from build123d import *

# Parameters (mm, degrees)
BOSS_EXTRUDE1_DEPTH   = 12.7
BOSS_EXTRUDE1_2_DEPTH = 12.7
BOSS_EXTRUDE2_REACH   = 26.909
CUT_EXTRUDE2_REACH    = 19.991
FILLET1_R             = 6.35
FILLET3_R             = 0.5


with BuildPart() as part:
    # Sketch1 → Boss-Extrude1 (new body)
    with BuildSketch(Plane(origin=(0, 0, 0), x_dir=(0, 0, -1), z_dir=(1, 0, 0))):
        with BuildLine():
            Line((9.214036359, -0.723419074), (9.52014781, -1.005011796))
            Line((9.52014781, -1.005011796), (9.931084378, -1.111282001))
            Line((9.931084378, -1.111282001), (9.790954894, -0.710625106))
            Line((9.790954894, -0.710625106), (9.214036359, -0.17991624))
            Line((9.214036359, -0.17991624), (8.098182028, -0.17991624))
            Line((8.098182028, -0.17991624), (8.098182028, -2.893389425))
            ThreePointArc((8.098182028, -2.893389425), (8.258948932, -3.437161263), (8.68955765, -3.80609207))
            Line((8.68955765, -3.80609207), (10.464036359, -4.600540583))
            Line((10.464036359, -4.600540583), (12.238515069, -3.80609207))
            ThreePointArc((12.238515069, -3.80609207), (12.669123787, -3.437161263), (12.829890691, -2.893389425))
            Line((12.829890691, -2.893389425), (12.829890691, -0.17991624))
            Line((12.829890691, -0.17991624), (11.714036359, -0.17991624))
            Line((11.714036359, -0.17991624), (11.714036359, -2.617334806))
            Line((11.714036359, -2.617334806), (9.214036359, -2.617334806))
            Line((9.214036359, -2.617334806), (9.214036359, -0.723419074))
        make_face()
    extrude(amount=BOSS_EXTRUDE1_DEPTH)


with BuildPart() as body_2:
    # Sketch1 → Boss-Extrude1 2 (new body)
    with BuildSketch(Plane(origin=(0, 0, 0), x_dir=(0, 0, -1), z_dir=(1, 0, 0))):
        with BuildLine():
            Line((-8.098182028, -0.17991624), (-9.214036359, -0.17991624))
            Line((-9.214036359, -0.17991624), (-9.790954894, -0.710625106))
            Line((-9.790954894, -0.710625106), (-9.931084378, -1.111282001))
            Line((-9.931084378, -1.111282001), (-9.52014781, -1.005011796))
            Line((-9.52014781, -1.005011796), (-9.214036359, -0.723419074))
            Line((-9.214036359, -0.723419074), (-9.214036359, -2.617334806))
            Line((-9.214036359, -2.617334806), (-11.714036359, -2.617334806))
            Line((-11.714036359, -2.617334806), (-11.714036359, -0.17991624))
            Line((-11.714036359, -0.17991624), (-12.829890691, -0.17991624))
            Line((-12.829890691, -0.17991624), (-12.829890691, -2.893389425))
            ThreePointArc((-12.829890691, -2.893389425), (-12.669123787, -3.437161263), (-12.238515069, -3.80609207))
            Line((-12.238515069, -3.80609207), (-10.464036359, -4.600540583))
            Line((-10.464036359, -4.600540583), (-8.68955765, -3.80609207))
            ThreePointArc((-8.68955765, -3.80609207), (-8.258948932, -3.437161263), (-8.098182028, -2.893389425))
            Line((-8.098182028, -2.893389425), (-8.098182028, -0.17991624))
        make_face()
    extrude(amount=BOSS_EXTRUDE1_2_DEPTH)

    # Sketch2 → Boss-Extrude2 (add, up to next)
    with BuildSketch(Plane.XY.offset(-8.098182028), mode=Mode.PRIVATE) as boss_extrude2_sk1:
        Polygon((5.47811731, -0.17991624), (7.387826905, -0.17991624), (7.387826905, -1.641579788), (6.432972108, -2.596434586), (5.47811731, -1.641579788), align=None)
    boss_extrude2_tool1 = extrude(boss_extrude2_sk1.sketch, amount=BOSS_EXTRUDE2_REACH, mode=Mode.PRIVATE) - body_2.part

    add(part.part)  # Boss-Extrude2 merges part
    add(boss_extrude2_tool1.solids().sort_by_distance((6.432972, -1.169053, -8.098182))[0])

    # Sketch5 → Loft4 section 0
    with BuildSketch(Plane(origin=(0, -0.17991624, 0), x_dir=(1, 0, 0), z_dir=(0, 1, 0))):
        with BuildLine():
            Line((7.387826905, 4.313769845), (7.387826905, -4.313769845))
            Line((7.387826905, -4.313769845), (6.432972108, -5.268624642))
            Line((6.432972108, -5.268624642), (5.47811731, -4.313769845))
            Line((5.47811731, -4.313769845), (5.47811731, 4.313769845))
            Line((5.47811731, 4.313769845), (6.432972108, 5.268624642))
            Line((6.432972108, 5.268624642), (7.387826905, 4.313769845))
        make_face()
    # Sketch6 → Loft4 section 1
    with BuildSketch(Plane(origin=(0, -10.33991624, 0), x_dir=(1, 0, 0), z_dir=(0, 1, 0))):
        with BuildLine():
            Line((6.432972108, -1.017808112), (5.47811731, -0.062953314))
            Line((5.47811731, -0.062953314), (5.47811731, 0.062953314))
            Line((5.47811731, 0.062953314), (6.432972108, 1.017808112))
            Line((6.432972108, 1.017808112), (7.387826905, 0.062953314))
            Line((7.387826905, 0.062953314), (7.387826905, -0.062953314))
            Line((7.387826905, -0.062953314), (6.432972108, -1.017808112))
        make_face()
    loft()

    # Sketch4 → Cut-Extrude2 (cut, up to next)
    with BuildSketch(Plane.ZY.offset(-5.47811731), mode=Mode.PRIVATE) as cut_extrude2_sk1:
        with BuildLine():
            Line((0.863271786, -3.536832517), (0.455999977, -3.536832517))
            Line((0.455999977, -3.536832517), (0.455999977, -3.028389789))
            Line((0.455999977, -3.028389789), (-0.455999977, -3.028389789))
            Line((-0.455999977, -3.028389789), (-0.455999977, -3.536832517))
            Line((-0.455999977, -3.536832517), (-0.863271786, -3.536832517))
            ThreePointArc((-0.863271786, -3.536832517), (-1.248147381, -3.717660499), (-1.354637866, -4.129349409))
            Line((-1.354637866, -4.129349409), (-0.455999977, -8.902101345))
            Line((-0.455999977, -8.902101345), (-0.455999977, -12.003161214))
            Line((-0.455999977, -12.003161214), (0.455999977, -12.003161214))
            Line((0.455999977, -12.003161214), (0.455999977, -8.902101345))
            Line((0.455999977, -8.902101345), (1.354637866, -4.129349409))
            ThreePointArc((1.354637866, -4.129349409), (1.248147381, -3.717660499), (0.863271786, -3.536832517))
        make_face()
    cut_extrude2_tool1 = extrude(cut_extrude2_sk1.sketch, amount=-CUT_EXTRUDE2_REACH, mode=Mode.PRIVATE) & body_2.part
    add(cut_extrude2_tool1.solids().sort_by_distance((5.478117, -6.679281, 0))[0], mode=Mode.SUBTRACT)

    # Fillet1
    # the kernel refuses this fillet: 6.35 mm, written as the material it adds along each edge
    with BuildSketch(Plane(origin=(11.918265355, 2.888858661, -1.067268312), x_dir=(0.268949751125616, 0.268949751125617, -0.9248416419792839), z_dir=(-0.6539617965672524, -0.6539617965672533, -0.3803523856387155))) as fillet1_piece_1_section:
        with BuildLine():
            CenterArc((FILLET1_R * 0.436389328948, FILLET1_R), FILLET1_R, 222.8481144, 47.1518856)
            Line((-FILLET1_R * 0.296769712888, FILLET1_R * 0.319942782278), (0, 0))
            Line((0, 0), (FILLET1_R * 0.436389328948, 0))
        make_face()
    fillet1_piece_1 = extrude(amount=15.315469113, mode=Mode.PRIVATE)
    fillet1_piece_1 = split(fillet1_piece_1, bisect_by=Plane(origin=(7.387826905, 2.888858661, -1.067268312), z_dir=(-1, 0, 0)), keep=Keep.TOP, mode=Mode.PRIVATE)
    fillet1_piece_1 = fillet1_piece_1 - Plane(origin=(0.404018799, -5.547737398, -6.35885034), x_dir=(0.7071067811865474, 0.7071067811865479, 0), z_dir=(0.6539617965672531, -0.6539617965672526, -0.38035238563871554)) * Cylinder(6.35, 42, mode=Mode.PRIVATE)
    add(fillet1_piece_1)
    with BuildSketch(Plane(origin=(10.963410557, -7.126873035, -6.892543527), x_dir=(-0.26894975112561653, 0.26894975112561653, -0.9248416419792839), z_dir=(-0.6539617965672532, 0.6539617965672525, 0.38035238563871554))) as fillet1_piece_2_section:
        with BuildLine():
            CenterArc((FILLET1_R * 0.436389328948, FILLET1_R), FILLET1_R, 222.8481144, 47.1518856)
            Line((-FILLET1_R * 0.296769712888, FILLET1_R * 0.319942782278), (0, 0))
            Line((0, 0), (FILLET1_R * 0.436389328948, 0))
        make_face()
    fillet1_piece_2 = extrude(amount=15.315469113, mode=Mode.PRIVATE)
    fillet1_piece_2 = split(fillet1_piece_2, bisect_by=Plane(origin=(5.47811731, -7.126873035, -6.892543527), z_dir=(1, 0, 0)), keep=Keep.TOP, mode=Mode.PRIVATE)
    fillet1_piece_2 = fillet1_piece_2 - Plane(origin=(11.012970172, -6.996692643, -7.201580889), x_dir=(-0.707106781186548, 0.7071067811865471, 0), z_dir=(0.6539617965672524, 0.6539617965672532, 0.38035238563871543)) * Cylinder(6.35, 42, mode=Mode.PRIVATE)
    add(fillet1_piece_2)
    with BuildSketch(Plane(origin=(1.902533659, -7.126873035, 6.892543527), x_dir=(0.33552051071253974, -0.7013229496273355, -0.6289452338774898), z_dir=(0.6539617965672524, 0.6539617965672533, -0.3803523856387155))) as fillet1_piece_3_section:
        with BuildLine():
            CenterArc((FILLET1_R * 0.436389328948, -FILLET1_R), FILLET1_R, 90, 47.1518856)
            Line((-FILLET1_R * 0.296769712888, -FILLET1_R * 0.319942782278), (0, 0))
            Line((0, 0), (FILLET1_R * 0.436389328948, 0))
        make_face()
    fillet1_piece_3 = extrude(amount=15.315469113, mode=Mode.PRIVATE)
    fillet1_piece_3 = split(fillet1_piece_3, bisect_by=Plane(origin=(7.387826905, -7.126873035, 6.892543527), z_dir=(-1, 0, 0)), keep=Keep.TOP, mode=Mode.PRIVATE)
    fillet1_piece_3 = fillet1_piece_3 - Plane(origin=(1.852974044, -6.996692643, 7.201580889), x_dir=(0.7071067811865474, 0.7071067811865479, 0), z_dir=(-0.6539617965672531, 0.6539617965672526, -0.38035238563871554)) * Cylinder(6.35, 42, mode=Mode.PRIVATE)
    add(fillet1_piece_3)
    with BuildSketch(Plane(origin=(0.947678861, 2.888858661, 1.067268313), x_dir=(-0.26894975112561653, 0.26894975112561653, 0.9248416419792839), z_dir=(0.6539617965672532, -0.6539617965672525, 0.38035238563871554))) as fillet1_piece_4_section:
        with BuildLine():
            CenterArc((FILLET1_R * 0.436389328948, FILLET1_R), FILLET1_R, 222.8481144, 47.1518856)
            Line((-FILLET1_R * 0.296769712888, FILLET1_R * 0.319942782278), (0, 0))
            Line((0, 0), (FILLET1_R * 0.436389328948, 0))
        make_face()
    fillet1_piece_4 = extrude(amount=15.315469113, mode=Mode.PRIVATE)
    fillet1_piece_4 = split(fillet1_piece_4, bisect_by=Plane(origin=(5.47811731, 2.888858661, 1.067268313), z_dir=(1, 0, 0)), keep=Keep.TOP, mode=Mode.PRIVATE)
    fillet1_piece_4 = fillet1_piece_4 - Plane(origin=(12.461925417, -5.547737398, 6.35885034), x_dir=(-0.6780560120828721, 0.28369012840869895, -0.6780560120828721), z_dir=(-0.6539617965672524, -0.6539617965672532, 0.3803523856387155)) * Cylinder(6.35, 42, mode=Mode.PRIVATE)
    add(fillet1_piece_4)

    # Fillet3
    fillet3_edges = [body_2.edges().sort_by_distance(p)[0] for p in [
        (7.387826905, -0.910748014, 8.098182028),
        (5.47811731, -0.910748014, 8.098182028),
        (7.387826905, -0.910748014, -8.098182028),
        (5.47811731, -0.910748014, -8.098182028),
    ]]
    fillet(fillet3_edges, radius=FILLET3_R)


solid = body_2.part
Build history of the part. All positions in model axes, mm. A direction names the side the tool comes from. Coordinates: 2 decimals unless noted, no trailing zeros. Use CSV: the item, a comma, the result in double quotes. Start each with the question number.
Q1. Pull direction Y, two halves, no side cores. Call faces 5 (the flat face through (6.3, -2.7, -8.098)), 6 (the flat face through (6.26, -4.2, 11.36)), 7 (the flat face through (6.42, -6.482, -0.912)), 8 (the flat face through (6, -2.617, 10)): released by +Y, released by -Y, zero draft, split by the parting line, or undercut.
Q2. Cut at B-B, the plane y = -2. State how many separate pieces and enclosed holes the cut face has, then the cut area to 3 significant figures.
Q3. 3-axis set-ups, long thin cutter, end or side, ignore diameter. For faces 1 (the cylindrical face through (6.26, -3.44, 8.26)), 2 (the flat face through (7.388, -2, 0)), 3 (the flat face through (6, -1, 11.714)), 4 (the flat face through (6, -2, 9.214)): which of +Z, -Z, +X, -X, +Y, -Y reach the whole face in a straight line?
Q4. Drill centre lines: probe 1 along Z at (x, y) = (6.25, -1.5); probe 2 along Z at (x, y) = (0.5, -2); probe 3 along Y at (x, z) = (9.25, 9.5). Where is each one in solid material? Low to high.
Q5. Flat gauge pins, fed straight in: pin 1 Ø3 at (x, z) = (4, -10.5) entering from +Y; pin 2 Ø0.7 at (x, y) = (6.5, -10) entering from +Z; pin 3 Ø2 at (x, z) = (6, 10.5) entering from +Y. Where does each tip first touch, or does it go through?
Checked values:
1,face 5,"zero draft"
1,face 6,"released by -Y"
1,face 7,"undercut"
1,face 8,"undercut"
2,separate pieces,"3"
2,enclosed holes,"0"
2,area,"84.0 mm²"
3,face 1,"+X, -X, -Y"
3,face 2,"+X, +Y, -Y"
3,face 3,"+X, -X, +Y"
3,face 4,"+X, -X"
4,probe 1,"z = -12.83 to -11.71, -9.21 to 9.21, 11.71 to 12.83"
4,probe 2,"z = -12.83 to -11.71, -9.21 to -8.1, 8.1 to 9.21, 11.71 to 12.83"
4,probe 3,"y = -4.17 to -2.62, -0.99 to -0.44"
5,pin 1,"stops at y = -0.18"
5,pin 2,"stops at z = 1.3"
5,pin 3,"stops at y = -0.44"
